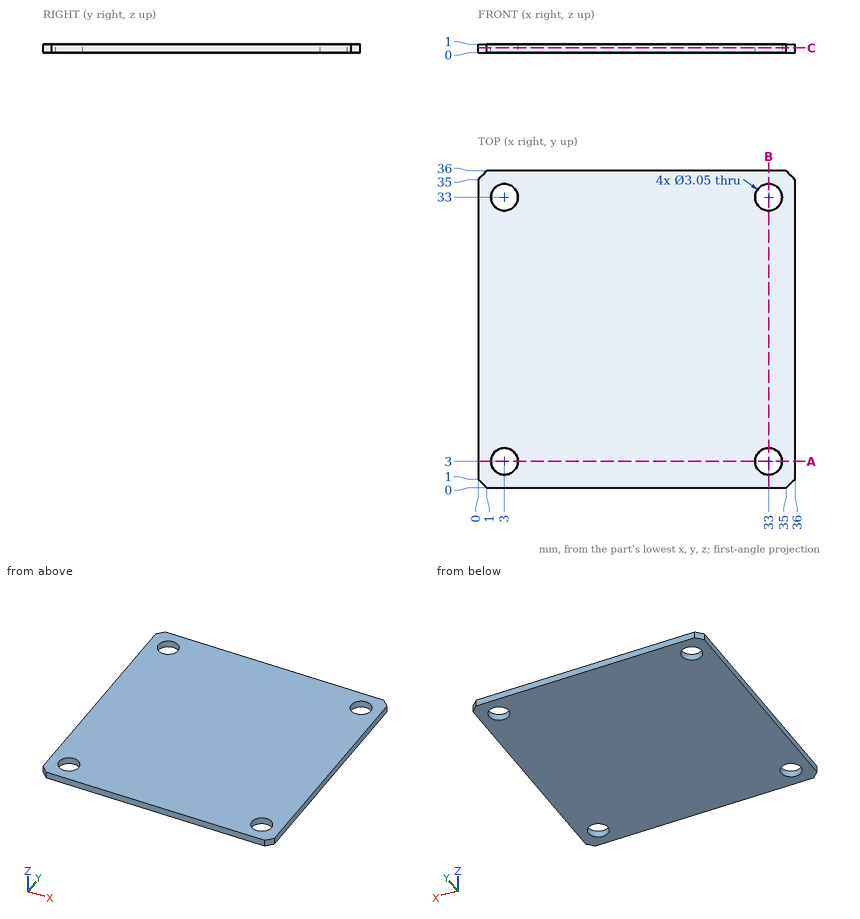
Could you check a few things on this drawing? It's one solid part, dimensions in mm from its lowest x, y, z. Coordinates: 2 decimals unless noted, no trailing zeros. Loops run counter-clockwise (first coordinate to the right, second up) from the corner with the lowest first, then second, coordinate; pieces in that order, holes last.
1. Imagine slicing it at A-A (y = 3). Please give me the cut outline in (x, z) (3 decimals), and give its area (3 significant figures).
2. Imagine slicing it at C-C (z = 0.55). Please give me the cut outline in (x, y) (3 decimals), and give its area (3 significant figures).
3. For P1, Ø2.5, axis at x = 33, y = 3, coming from the +Z side, with a flat end and sliding along its axis, tell me the tip position at first contact or that it passes through.
4. I need wall thicknesses on L1, parallel to X at y = 3, z = 0.4 (3 decimals); L2, parallel to X at y = 3.5, z = 0.9. Which ranges of each line are inside material? Lowest first, please.
Computed values:
1. outline: (0, 0) - (1.475, 0) - (1.475, 1) - (0, 1) - close; (4.525, 0) - (31.475, 0) - (31.475, 1) - (4.525, 1) - close; (34.525, 0) - (36, 0) - (36, 1) - (34.525, 1) - close
1. area: 29.9 mm2
2. outline: (0, 1) - (1, 0) - (35, 0) - (36, 1) - (36, 35) - (35, 36) - (1, 36) - (0, 35) - close; hole circle Ø3.05 at (3, 3); hole circle Ø3.05 at (3, 33); hole circle Ø3.05 at (33, 3); hole circle Ø3.05 at (33, 33)
2. area: 1,260 mm2
3. P1: passes through
4. L1: x = 0 to 1.475, 4.525 to 31.475, 34.525 to 36
4. L2: x = 0 to 1.56, 4.44 to 31.56, 34.44 to 36
